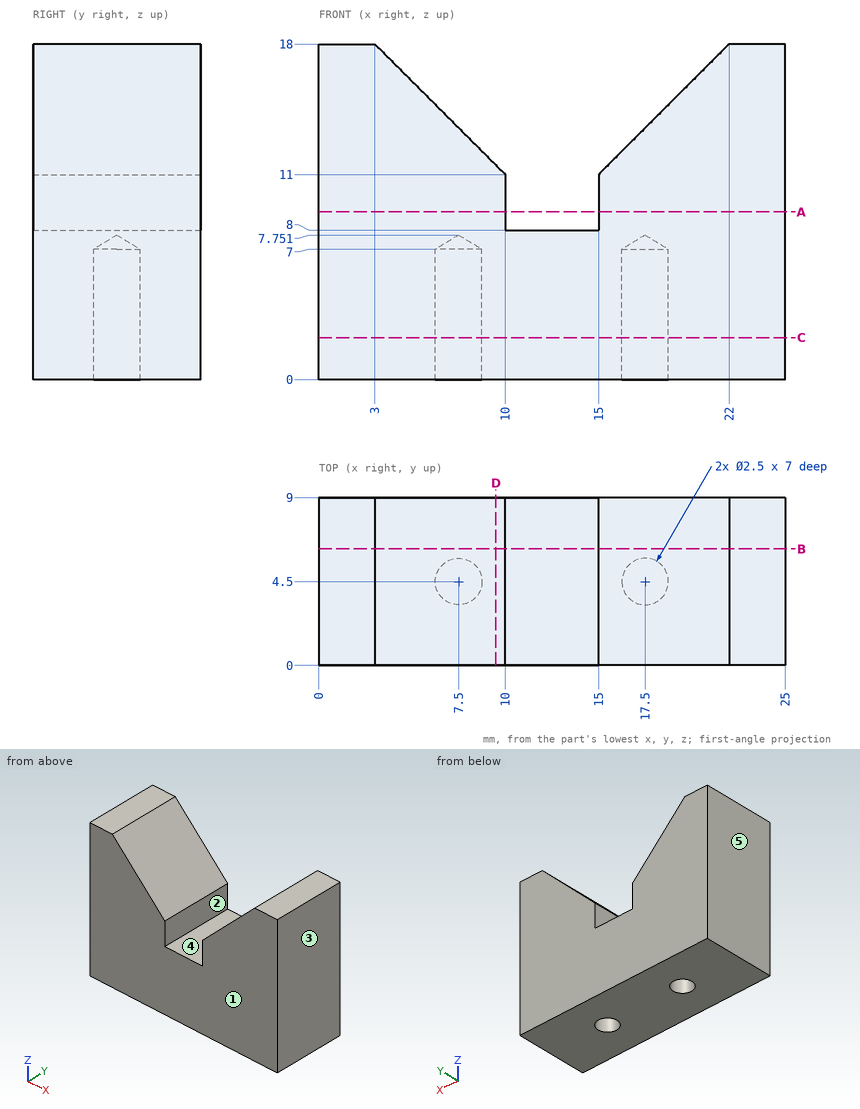
Verification items for this drawing (mm, ordinates from the low corner). A direction names the side the tool comes from. Coordinates: 2 decimals unless noted, no trailing zeros. Order: outer loops, then holes, each group sorted by start corner. A loop starts at its lowest first (then second) coordinate and runs counter-clockwise, first axis right, second up.
Q1. Depth check by flat-ended pin: pin 1 Ø3 at (x, y) = (7.5, 4.5) entering from -Z; pin 2 Ø2 at (x, y) = (17.5, 4.5) entering from +Z; pin 3 Ø1 at (x, y) = (15, 8) entering from +Z. Enter the tip coordinate at first touch or a pass-through.
Reply:
pin 1: stops at z = 0
pin 2: stops at z = 14.5
pin 3: stops at z = 11.5
Q2. Sectioned sample at A-A on z = 9. Record the cut outline in (x, y), and give its area (3 significant figures).
Reply:
outline: (0, 0) - (10, 0) - (10, 9) - (0, 9) - close; (15, 0) - (25, 0) - (25, 9) - (15, 9) - close
area: 180 mm2
Q3. Sectioned sample at C-C on z = 2.25. Record the cut outline in (x, y).
Reply:
outline: (0, 0) - (25, 0) - (25, 9) - (0, 9) - close; hole circle Ø2.5 at (7.5, 4.5); hole circle Ø2.5 at (17.5, 4.5)
Q4. Draft check along X on the marked faces 1, 2 and 3. Enter one of: released by +X, released by -X, zero draft, split by the parting line, or undercut.
Reply:
face 1: zero draft
face 2: undercut
face 3: released by +X
Q5. Sectioned sample at D-D on x = 9.5. Record the cut outline in (y, z).
Reply:
outline: (0, 0) - (9, 0) - (9, 11.5) - (0, 11.5) - close
Q6. Thickness scan on probe 1 along X at (y, z) = (4.5, 3.75); probe 2 along Y at (x, z) = (17.5, 4); probe 3 along Z at (x, y) = (13.75, 3.75). Record the ranges inside material, lowest first.
Reply:
probe 1: x = 0 to 6.25, 8.75 to 16.25, 18.75 to 25
probe 2: y = 0 to 3.25, 5.75 to 9
probe 3: z = 0 to 8
Q7. Sectioned sample at B-B on y = 6.25. Record the cut outline in (x, z).
Reply:
outline: (0, 0) - (25, 0) - (25, 18) - (22, 18) - (15, 11) - (15, 8) - (10, 8) - (10, 11) - (3, 18) - (0, 18) - close
Q8. Tool access check on the marked faces 4 and 5. Record the directions out of +Z, -Z, +X, -X, +Y, -Y that give a thin tool (end or side, any length) a straight path to the whole face; none if there is none.
Reply:
face 4: +Z, +Y, -Y
face 5: +Z, -Z, -X, +Y, -Y
